For this review, take the finished solid that the model builds, in its own axes (mm). Face numbers are marked on the shaded views. A direction names the side the tool comes from. Round coordinates to 2 decimals unless told otherwise and drop trailing zeros. Loops run counter-clockwise (first coordinate to the right, second up) from the corner with the lowest first, then second, coordinate; pieces in that order, holes last.
```python
from build123d import *

# Parameters (mm, degrees)
SKETCH1_W           = 125
SKETCH1_H           = 94
BOSS_EXTRUDE1_DEPTH = 40
SKETCH2_W           = 114.291192295
SKETCH2_H           = 86
CUT_EXTRUDE1_DEPTH  = 30
CUT_EXTRUDE2_START  = 61.163706
SKETCH3_W           = 13
SKETCH3_H           = 15
CUT_EXTRUDE2_DEPTH  = 10
SKETCH4_R           = 4
BOSS_EXTRUDE2_DEPTH = 20
SKETCH5_R           = 2
CUT_EXTRUDE3_DEPTH  = 15
CUT_EXTRUDE4_START  = -38.836294
SKETCH6_W           = 45
SKETCH6_H           = 12
CUT_EXTRUDE4_DEPTH  = 10
SKETCH7_W           = 60
SKETCH7_H           = 60
BOSS_EXTRUDE3_DEPTH = 40
SKETCH8_W           = 62.296403185
SKETCH8_H           = 47.840676856
CUT_EXTRUDE5_DEPTH  = 30


with BuildPart() as part:
    # Sketch1 → Boss-Extrude1 (new body)
    with BuildSketch(Plane(origin=(0, 0, 0), x_dir=(1, 0, 0), z_dir=(0, 1, 0))):
        with Locations((11.421319797, -14.163705584)):
            Rectangle(SKETCH1_W, SKETCH1_H)
    extrude(amount=BOSS_EXTRUDE1_DEPTH)

    # Sketch2 → Cut-Extrude1 (cut)
    with BuildSketch(Plane(origin=(0, 0, 0), x_dir=(1, 0, 0), z_dir=(0, 1, 0))):
        with Locations((12.77572365, -14.163705584)):
            Rectangle(SKETCH2_W, SKETCH2_H)
    extrude(amount=CUT_EXTRUDE1_DEPTH, mode=Mode.SUBTRACT)

    # Sketch3 → Cut-Extrude2 (cut)
    with BuildSketch(Plane.XY.offset(CUT_EXTRUDE2_START)):
        with Locations((-17.578680203, 15.5)):
            Rectangle(SKETCH3_W, SKETCH3_H)
        with Locations((40.421319797, 15.5)):
            Rectangle(SKETCH3_W, SKETCH3_H)
    extrude(amount=-CUT_EXTRUDE2_DEPTH, mode=Mode.SUBTRACT)

    # Sketch4 → Boss-Extrude2 (add)
    with BuildSketch(Plane(origin=(0, 0, 0), x_dir=(1, 0, 0), z_dir=(0, 1, 0))):
        with Locations((-43.22295396, -55.91654856)):
            Circle(SKETCH4_R)
        with Locations((68.117960644, -55.91654856)):
            Circle(SKETCH4_R)
        with Locations((68.117960644, 26.819499734)):
            Circle(SKETCH4_R)
        with Locations((-43.22295396, 26.819499734)):
            Circle(SKETCH4_R)
    extrude(amount=BOSS_EXTRUDE2_DEPTH)

    # Sketch5 → Cut-Extrude3 (cut)
    with BuildSketch(Plane(origin=(0, 0, 0), x_dir=(1, 0, 0), z_dir=(0, 1, 0))):
        with Locations(Location((-43.864318676, -56.044821503, 0), (0, 0, 270))):
            Circle(SKETCH5_R)
        with Locations(Location((67.989687701, -56.044821503, 0), (0, 0, 270))):
            Circle(SKETCH5_R)
        with Locations(Location((68.117960644, 26.819499734, 0), (0, 0, 270))):
            Circle(SKETCH5_R)
        with Locations(Location((-43.864318676, 26.819499734, 0), (0, 0, 270))):
            Circle(SKETCH5_R)
    extrude(amount=CUT_EXTRUDE3_DEPTH, mode=Mode.SUBTRACT)

    # Sketch6 → Cut-Extrude4 (cut)
    with BuildSketch(Plane.XY.offset(CUT_EXTRUDE4_START)):
        with Locations((11.421319797, 20)):
            Rectangle(SKETCH6_W, SKETCH6_H)
    extrude(amount=CUT_EXTRUDE4_DEPTH, mode=Mode.SUBTRACT)

    # Sketch7 → Boss-Extrude3 (add)
    with BuildSketch(Plane(origin=(0, 0, 0), x_dir=(1, 0, 0), z_dir=(0, 1, 0))):
        with Locations((-81.078680203, -17.322261373)):
            Rectangle(SKETCH7_W, SKETCH7_H)
    extrude(amount=BOSS_EXTRUDE3_DEPTH)

    # Sketch8 → Cut-Extrude5 (cut)
    with BuildSketch(Plane(origin=(0, 0, 0), x_dir=(1, 0, 0), z_dir=(0, 1, 0))):
        with Locations((-75.518074091, -18.055506677)):
            Rectangle(SKETCH8_W, SKETCH8_H)
    extrude(amount=CUT_EXTRUDE5_DEPTH, mode=Mode.SUBTRACT)


solid = part.part
```
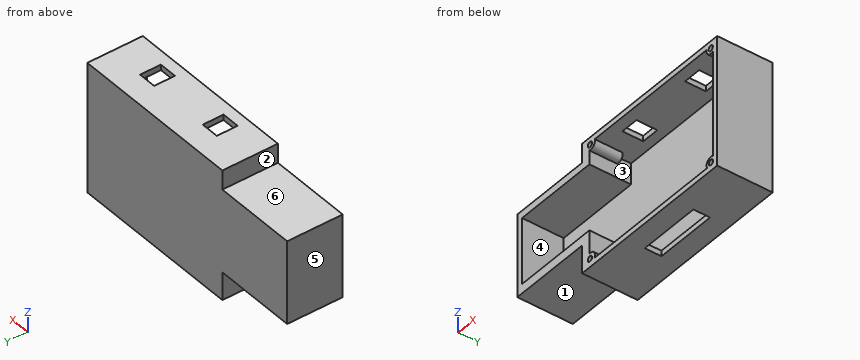
(1) Add section A-A (x = -14). Give the boundary of the cut face in (y, z), plus the area to 3 significant figures.
(2) The part is to be moulded in two halves that separate along X. For the marked faces 4, 5 and 6, say which applies: pulls with the +X half, pulls with the -X half, needs draft (parallel to the pull), parting line crosses it, or undercut.
(3) Add section B-B (z = 20). Give the boundary of the cut face in (x, y).
(4) For L1, parallel to X at y = 8, z = -27; L2, parallel to X at y = 10.5, z = 41; L3, parallel to Z at x = -52.5, y = 20, list the stretches that pass through material, from the lowest coordinate up.
(5) Add section C-C (y = 36.5). Give the boundary of the cut face in (x, z).
(6) For the marked faces 1, 2 and 3, list the 3-axis set-ups (+Z, -Z, +X, -X, +Y, -Y) from which the entire face can be reached by the end or side of a thin tool; tool diameter is ignored.
(7) Insertion check: pin 1 Ø4 at (x, z) = (-31, 49.5) entering from -Y; pin 2 Ø3 at (x, z) = (69, 56.5) entering from -Y; pin 3 Ø6 at (x, y) = (-76, 18) entering from +Z; pin 4 Ø4.5 at (y, z) = (17, 58.5) entering from -X. Each pin has a flat end and moves straight along its axis. Give the tip position at first contact, or say it passes through.
Outcome:
1. outline: (0, -32.84) - (40, -32.84) - (40, 61.16) - (23, 61.16) - (23, 57.16) - (30, 57.16) - (30, -28.84) - (0, -28.84) - close; (0, 57.16) - (8, 57.16) - (8, 61.16) - (0, 61.16) - close
1. area: 1,120 mm2
2. face 4: undercut
2. face 5: pulls with the -X half
2. face 6: needs draft
3. outline: (-111.08, 0) - (-106.67, 0) - (-106.67, 30) - (69.92, 30) - (69.92, 0) - (73.92, 0) - (73.92, 40) - (-111.08, 40) - close
4. L1: x = -51.08 to -45.86, -41.87 to -39.23, 64.12 to 66.13, 70.11 to 73.92
4. L2: x = -111.08 to -106.67, 69.92 to 73.92
4. L3: z = -12.68 to -5.86, 41.98 to 47.32
5. outline: (-111.08, -12.68) - (-51.08, -12.68) - (-51.08, -32.84) - (73.92, -32.84) - (73.92, 61.16) - (-51.08, 61.16) - (-51.08, 47.32) - (-111.08, 47.32) - close
6. face 1: -Z, -X, +Y, -Y
6. face 2: +Z, -X, +Y, -Y
6. face 3: none
7. pin 1: stops at y = 30
7. pin 2: stops at y = 0
7. pin 3: stops at z = 47.32
7. pin 4: stops at x = -51.08
